Part model, mm, in its own coordinate system. Face numbers are marked on the shaded views. Coordinates: 2 decimals unless noted, no trailing zeros. Loops run counter-clockwise (first coordinate to the right, second up) from the corner with the lowest first, then second, coordinate; pieces in that order, holes last. Notation, with made-up numbers: (-20, 25.25) - (25, 25.25) arc R14 ccw to (25, 52.25) - close; hole circle Ø9 at (-24.75, 32). An arc over 180 degrees is marked (long way). Use a Markdown table: item, result. Add a question column.
1. Band-saw the part on A-A, the plane x = 0. Give the cut face in (y, z).
2. Band-saw the part on C-C, the plane x = -3.8. Give the cut face in (y, z), plus the area to 3 significant figures.
3. Wall check: probe 1 along Z at (x, y) = (-4.25, -3); probe 2 along Y at (x, z) = (0, 6.2); probe 3 along X at (y, z) = (5, 6.5). Give the ranges that are in metal, low to high. Write a range as [from, to].
4. Band-saw the part on D-D, the plane y = 0.75. Give the cut face in (x, z), plus the area to 3 significant figures.
5. Pull direction X, two halves, no side cores. Call the marked faces 1, 2 and 3: pulls with the +X half, pulls with the -X half, needs draft (parallel to the pull), parting line crosses it, or undercut.
6. Drop flat-ended pins along their axis: pin 1 (1.5 mm diameter, centred on y = -4.5, z = 0.5, fed in from +X); pin 2 (1 mm diameter, centred on y = 1, z = 4.5, fed in from +X); pin 3 (3.5 mm diameter, centred on x = -1.5, y = -3, fed in from -Z). Give the stop position or say it passes through.
7. Band-saw the part on B-B, the plane y = 2. Give the cut face in (x, z), plus the area to 3 significant figures.
from build123d import *

# Parameters (mm, degrees)
SKETCH1_R           = 6
BOSS_EXTRUDE1_DEPTH = 7.5
SKETCH2_R           = 0.3
BOSS_EXTRUDE2_DEPTH = 2.5
SKETCH3_R           = 1.25
CUT_EXTRUDE1_DEPTH  = 1.8
SKETCH4_R           = 5.7
CUT_EXTRUDE2_DEPTH  = 1.5
SKETCH5_R           = 0.5
CUT_EXTRUDE3_DEPTH  = 0.1
SKETCH6_W           = 0.35
SKETCH6_H           = 0.1
SKETCH6_W_2         = 0.1
SKETCH6_H_2         = 0.35
BOSS_EXTRUDE3_DEPTH = 0.1


with BuildPart() as part:
    # Sketch1 → Boss-Extrude1 (new body)
    with BuildSketch(Plane.XY):
        Circle(SKETCH1_R)
    extrude(amount=BOSS_EXTRUDE1_DEPTH)

    # Sketch2 → Boss-Extrude2 (add)
    with BuildSketch(Plane(origin=(0, 0, 0), x_dir=(-1, 0, 0), z_dir=(0, 0, -1))):
        with Locations(Location((3.8, 0, 0), (0, 0, 180))):
            Circle(SKETCH2_R)
        with Locations(Location((-3.8, 0, 0), (0, 0, 180))):
            Circle(SKETCH2_R)
    extrude(amount=BOSS_EXTRUDE2_DEPTH)

    # Sketch3 → Cut-Extrude1 (cut)
    with BuildSketch(Plane.XY.offset(7.5)):
        Circle(SKETCH3_R)
    extrude(amount=-CUT_EXTRUDE1_DEPTH, mode=Mode.SUBTRACT)

    # Sketch4 → Cut-Extrude2 (cut)
    with BuildSketch(Plane.XY.offset(5.7)):
        Circle(SKETCH4_R)
    extrude(amount=CUT_EXTRUDE2_DEPTH, mode=Mode.SUBTRACT)

    # Sketch5 → Cut-Extrude3 (cut)
    with BuildSketch(Plane.XY.offset(7.5)):
        with Locations((3.8, 0)):
            Circle(SKETCH5_R)
    extrude(amount=-CUT_EXTRUDE3_DEPTH, mode=Mode.SUBTRACT)

    # Sketch6 → Boss-Extrude3 (add)
    with BuildSketch(Plane.XY.offset(7.4)):
        with Locations((4.025, 0)):
            Rectangle(SKETCH6_W, SKETCH6_H)
        with Locations((3.575, 0)):
            Rectangle(SKETCH6_W, SKETCH6_H)
        with Locations((3.8, 0.225)):
            Rectangle(SKETCH6_W_2, SKETCH6_H_2)
        with Locations((3.8, -0.225)):
            Rectangle(SKETCH6_W_2, SKETCH6_H_2)
        with Locations((3.8, 0)):
            Rectangle(SKETCH6_W_2, SKETCH6_H)
    extrude(amount=BOSS_EXTRUDE3_DEPTH)


solid = part.part
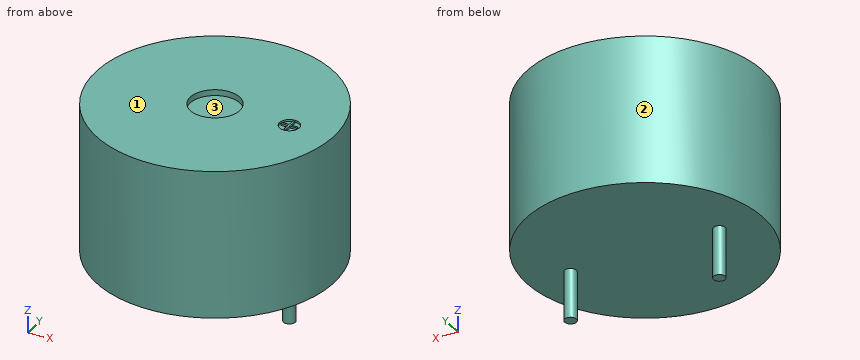
Geometry check:
| question | item | result |
|---|---|---|
| 1 | outline | (-6, 0) - (6, 0) - (6, 7.5) - (1.25, 7.5) - (1.25, 7.2) - (5.7, 7.2) - (5.7, 5.7) - (-5.7, 5.7) - (-5.7, 7.2) - (-1.25, 7.2) - (-1.25, 7.5) - (-6, 7.5) - close |
| 2 | outline | (-4.64, 0) - (-0.3, 0) - (-0.3, -2.5) - (0.3, -2.5) - (0.3, 0) - (4.64, 0) - (4.64, 7.5) - (-4.64, 7.5) - close; hole (-4.25, 5.7) - (4.25, 5.7) - (4.25, 7.2) - (-4.25, 7.2) - close |
| 2 | area | 58.4 mm^2 |
| 3 | probe 1 | z = [0, 5.7], [7.2, 7.5] |
| 3 | probe 2 | y = [-6, -5.7], [5.7, 6] |
| 3 | probe 3 | x = [-3.32, -2.74], [2.74, 3.32] |
| 4 | outline | (-5.95, 0) - (5.95, 0) - (5.95, 7.5) - (1, 7.5) - (1, 7.2) - (5.65, 7.2) - (5.65, 5.7) - (-5.65, 5.7) - (-5.65, 7.2) - (-1, 7.2) - (-1, 7.5) - (-5.95, 7.5) - close |
| 4 | area | 71.7 mm^2 |
| 5 | face 1 | needs draft |
| 5 | face 2 | parting line crosses it |
| 5 | face 3 | undercut |
| 6 | pin 1 | stops at x = 4.68 |
| 6 | pin 2 | stops at x = 5.98 |
| 6 | pin 3 | stops at z = 0 |
| 7 | outline | (-5.66, 0) - (5.66, 0) - (5.66, 7.5) - (-5.66, 7.5) - close; hole (-5.34, 5.7) - (5.34, 5.7) - (5.34, 7.2) - (-5.34, 7.2) - close |
| 7 | area | 68.8 mm^2 |
